Part model, mm, in its own coordinate system. Face numbers are marked on the shaded views. Round coordinates to 2 decimals unless told otherwise and drop trailing zeros. Write each loop counter-clockwise with the first axis right and the second up, starting at its lowest first coordinate (ties: lowest second). Pieces come first, ordered by that corner, then holes. Notation, with made-up numbers: M -36,13 L -27,13 A20 cw -27,43 Z; hole C 62.25,37.25 d1. An arc over 180 degrees is marked long. One line per question, with ' | ' between items. Start each with the question number.
1) Drop flat-ended pins along their axis: pin 1 Ø1 at (y, z) = (815.5, 175.5) entering from +X; pin 2 Ø6.5 at (x, y) = (0, 851.66) entering from +Z; pin 3 Ø8.5 at (x, y) = (-24.89, 774.36) entering from +Z. Give the stop position or say it passes through.
2) Saw through at C-C (y = 758). List the corners of the cut face in (x, z).
3) Wall check: probe 1 along Y at (x, z) = (0, 175); probe 2 along Y at (x, z) = (25.4, 173.05); probe 3 along X at (y, z) = (775, 176). Give the ranges that are in metal, low to high. Write a range as [from, to].
4) Saw through at A-A (x = 0). List the corners of the cut face in (y, z) (3 decimals), plus the area to 3 significant figures.
5) Mould opens along X. For the marked faces 1, 2, 3 and 4 say: pulls with the +X half, pulls with the -X half, needs draft (parallel to the pull), parting line crosses it, or undercut.
6) Saw through at D-D (z = 172.5). Give the number of separate pieces and of enclosed holes in the cut face, plus the area to 3 significant figures.
7) Saw through at B-B (x = 25.4). List the corners of the cut face in (y, z) (3 decimals).
```python
from build123d import *

# Parameters (mm, degrees)
SKETCH1_R           = 23.495
SKETCH1_R_2         = 3.175
SKETCH1_R_3         = 12.7
SKETCH1_R_4         = 1.984375
BOSS_EXTRUDE1_DEPTH = 6.35
FILLET1_R           = 4.7625
SKETCH2_R           = 3.175
CUT_EXTRUDE1_DEPTH  = 6.35
SKETCH2_3_R         = 3.175
BOSS_EXTRUDE2_DEPTH = 6.35
FILLET2_R           = 6.35
CHAMFER1_SIZE       = 1.905


with BuildPart() as part:
    # Sketch1 → Boss-Extrude1 (new body)
    with BuildSketch(Plane.XY.offset(171.45)):
        Polygon((38.1, 791.013640976), (31.430896424, 826.256140976), (0, 857.6870374), (-31.430896424, 826.256140976), (-38.1, 791.013640976), (-38.1, 734.498640976), (38.1, 734.498640976), align=None)
        with Locations((0, 762.756140976)):
            Circle(SKETCH1_R, mode=Mode.SUBTRACT)
        with Locations((-24.890610486, 774.362823262)):
            Circle(SKETCH1_R_2, mode=Mode.SUBTRACT)
        with Locations((24.890610486, 774.362823262)):
            Circle(SKETCH1_R_2, mode=Mode.SUBTRACT)
        with Locations((0, 826.256140976)):
            Circle(SKETCH1_R_3, mode=Mode.SUBTRACT)
        with Locations((-25.4, 826.256140976)):
            Circle(SKETCH1_R_4, mode=Mode.SUBTRACT)
        with Locations((0, 851.656140976)):
            Circle(SKETCH1_R_4, mode=Mode.SUBTRACT)
        with Locations((25.4, 826.256140976)):
            Circle(SKETCH1_R_4, mode=Mode.SUBTRACT)
        with Locations((0, 800.856140976)):
            Circle(SKETCH1_R_4, mode=Mode.SUBTRACT)
        with Locations((24.890610486, 751.14945869)):
            Circle(SKETCH1_R_2, mode=Mode.SUBTRACT)
        with Locations((-24.890610486, 751.14945869)):
            Circle(SKETCH1_R_2, mode=Mode.SUBTRACT)
    extrude(amount=BOSS_EXTRUDE1_DEPTH)

    # Fillet1
    fillet1_edges = [part.edges().sort_by_distance(p)[0] for p in [
        (0, 857.6870374, 174.625),
        (31.430896424, 826.256140976, 174.625),
        (38.1, 791.013640976, 174.625),
        (38.1, 734.498640976, 174.625),
        (-38.1, 734.498640976, 174.625),
        (-38.1, 791.013640976, 174.625),
        (-31.430896424, 826.256140976, 174.625),
    ]]
    fillet(fillet1_edges, radius=FILLET1_R)

    # Sketch2 → Cut-Extrude1 (cut)
    with BuildSketch(Plane.XY.offset(177.8)):
        with Locations((-27.94, 813.744260544)):
            Circle(SKETCH2_R)
    extrude(amount=-CUT_EXTRUDE1_DEPTH, mode=Mode.SUBTRACT)

    # Sketch2<3> → Boss-Extrude2 (add)
    # profile 1 of 2: a face of its own
    with BuildSketch(Plane.XY.offset(177.8)):
        with BuildLine():
            ThreePointArc((-34.612193634, 809.444756111), (-25.699088435, 806.129654736), (-20.0025, 813.744260544))
            ThreePointArc((-20.0025, 813.744260544), (-24.322344832, 820.809419943), (-32.579880116, 820.18440175))
            Line((-32.579880116, 820.18440175), (-34.612193634, 809.444756111))
        make_face()
        with Locations((-27.94, 813.744260544)):
            Circle(SKETCH2_3_R, mode=Mode.SUBTRACT)
    # profile 2 of 2: a face of its own
    with BuildSketch(Plane.XY.offset(177.8)):
        with BuildLine():
            Line((-34.612193634, 809.444756111), (-32.579880116, 820.18440175))
            ThreePointArc((-32.579880116, 820.18440175), (-35.739086501, 815.220118263), (-34.612193634, 809.444756111))
        make_face()
    extrude(amount=-BOSS_EXTRUDE2_DEPTH)

    # Fillet2
    fillet2_edges = [part.edges().sort_by_distance(p)[0] for p in [
        (-32.579880116, 820.18440175, 174.625),
        (-34.612193634, 809.444756111, 174.625),
    ]]
    fillet(fillet2_edges, radius=FILLET2_R)

    # Chamfer1
    chamfer1_edges = [part.edges().sort_by_distance(p)[0] for p in [
        (-27.384375, 826.256140976, 177.8),
        (-1.984375, 851.656140976, 177.8),
        (23.415625, 826.256140976, 177.8),
        (-1.984375, 800.856140976, 177.8),
    ]]
    chamfer(chamfer1_edges, length=CHAMFER1_SIZE)


solid = part.part
```
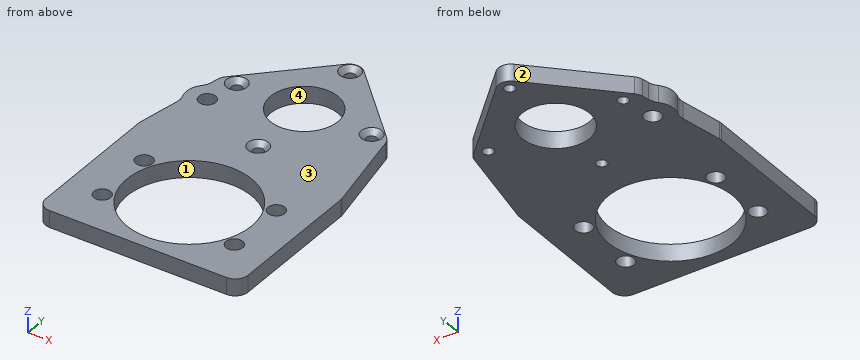
Answer key:
1) pin 1: stops at x = 33.56 | pin 2: stops at z = 177.16 | pin 3: stops at z = 177.8
2) outline: M -38.1,171.45 L -23.01,171.45 L -23.01,177.8 L -38.1,177.8 Z; M 23.01,171.45 L 38.1,171.45 L 38.1,177.8 L 23.01,177.8 Z
3) probe 1: y = [734.5, 739.26], [786.25, 798.87], [802.84, 813.56], [838.96, 849.67], [853.64, 855.71] | probe 2: y = [734.5, 748.02], [754.28, 771.23], [777.5, 824.27], [828.24, 832.29] | probe 3: x = [-38.1, -28], [-21.78, -20.05], [20.05, 21.78], [28, 38.1]
4) outline: M 734.499,171.45 L 739.261,171.45 L 739.261,177.8 L 734.499,177.8 Z; M 786.251,171.45 L 798.872,171.45 L 798.872,175.895 L 796.967,177.8 L 786.251,177.8 Z; M 802.841,171.45 L 813.556,171.45 L 813.556,177.8 L 804.746,177.8 L 802.841,175.895 Z; M 838.956,171.45 L 849.672,171.45 L 849.672,175.895 L 847.767,177.8 L 838.956,177.8 Z; M 853.641,171.45 L 855.714,171.45 L 855.714,177.8 L 855.546,177.8 L 853.641,175.895 Z | area: 252 mm2
5) face 1: undercut | face 2: pulls with the -X half | face 3: needs draft | face 4: undercut
6) separate pieces: 1 | enclosed holes: 11 | area: 5,300 mm2
7) outline: M 734.499,171.45 L 748.016,171.45 L 748.016,177.8 L 734.499,177.8 Z; M 754.283,171.45 L 771.229,171.45 L 771.229,177.8 L 754.283,177.8 Z; M 777.497,171.45 L 824.272,171.45 L 824.272,175.895 L 822.367,177.8 L 777.497,177.8 Z; M 828.241,171.45 L 832.287,171.45 L 832.287,177.8 L 830.146,177.8 L 828.241,175.895 Z
